Part model, mm, in its own coordinate system. Face numbers are marked on the shaded views. A direction names the side the tool comes from. Give positions to 0.01 mm unless a question says otherwise; leave off trailing zeros. Order: outer loops, then holes, each group sorted by start corner. A loop starts at its lowest first (then second) coordinate and runs counter-clockwise, first axis right, second up. Notation, with made-up numbers: (37.25, 53) - (84.25, 53) arc R23 cw to (84.25, 71) - close; hole circle Ø7 at (41, 11.5). An arc over 180 degrees is marked (long way). One line per item, written item: value.
```python
from build123d import *

# Parameters (mm, degrees)
BOSS_EXTRUDE1_DEPTH      = 30
SKETCH2_R                = 5
CUT_EXTRUDE1_DEPTH       = 30
BOSS_EXTRUDE2_DEPTH      = 10
BOSS_EXTRUDE2_DEPTH_BACK = 10
SKETCH4_W                = 159.060966422
SKETCH4_H                = 100
CUT_EXTRUDE2_DEPTH       = 55
CUT_EXTRUDE3_DEPTH       = 10
CUT_EXTRUDE3_DEPTH_BACK  = 5
SKETCH6_R                = 4.5
BOSS_EXTRUDE3_DEPTH      = 5


with BuildPart() as part:
    # Sketch1 → Boss-Extrude1 (new body)
    with BuildSketch(Plane(origin=(0, 0, 0), x_dir=(1, 0, 0), z_dir=(0, 1, 0))):
        with BuildLine():
            Line((2.5, 100), (0, 100))
            Line((0, 100), (0, 97.5))
            Line((0, 97.5), (0, 2.5))
            ThreePointArc((0, 2.5), (0.732233047, 0.732233047), (2.5, 0))
            Line((2.5, 0), (305, 0))
            ThreePointArc((305, 0), (315.606601718, 4.393398282), (320, 15))
            Line((320, 15), (320, 85))
            ThreePointArc((320, 85), (315.606601718, 95.606601718), (305, 100))
            Line((305, 100), (2.5, 100))
        make_face()
        with BuildLine():
            Line((20, 95), (300, 95))
            ThreePointArc((300, 95), (310.606601718, 90.606601718), (315, 80))
            Line((315, 80), (315, 20))
            ThreePointArc((315, 20), (310.606601718, 9.393398282), (300, 5))
            Line((300, 5), (20, 5))
            ThreePointArc((20, 5), (9.393398282, 9.393398282), (5, 20))
            Line((5, 20), (5, 80))
            ThreePointArc((5, 80), (9.393398282, 90.606601718), (20, 95))
        make_face(mode=Mode.SUBTRACT)
    extrude(amount=BOSS_EXTRUDE1_DEPTH)

    # Sketch2 → Cut-Extrude1 (cut)
    with BuildSketch(Plane(origin=(0, 0, 0), x_dir=(0, 0, -1), z_dir=(1, 0, 0))):
        with Locations((50, 3)):
            Circle(SKETCH2_R)
    extrude(amount=CUT_EXTRUDE1_DEPTH, mode=Mode.SUBTRACT)

    # Sketch3 → Boss-Extrude2 (add, two sides: drawn at the far end of the back side and taken through both)
    with BuildSketch(Plane(origin=(160, 0, 0), x_dir=(0, 0, -1), z_dir=(1, 0, 0)).offset(-BOSS_EXTRUDE2_DEPTH_BACK)):
        Polygon((5, 0), (5, 5), (7.5, 2.5), align=None)
        Polygon((95, 0), (95, 5), (92.5, 2.5), align=None)
    extrude(amount=BOSS_EXTRUDE2_DEPTH + BOSS_EXTRUDE2_DEPTH_BACK)

    # Sketch4 → Cut-Extrude2 (cut)
    with BuildSketch(Plane(origin=(0, 0, 0), x_dir=(1, 0, 0), z_dir=(0, 1, 0))):
        with Locations((249.530483211, 50)):
            Rectangle(SKETCH4_W, SKETCH4_H)
    extrude(amount=CUT_EXTRUDE2_DEPTH, mode=Mode.SUBTRACT)

    # Sketch5 → Cut-Extrude3 (cut, two sides: drawn at the far end of the back side and taken through both)
    with BuildSketch(Plane(origin=(160, 0, 0), x_dir=(0, 0, -1), z_dir=(1, 0, 0)).offset(-CUT_EXTRUDE3_DEPTH_BACK)):
        with BuildLine():
            ThreePointArc((3.5, 25), (3.207106781, 25.707106781), (2.5, 26))
            Line((2.5, 26), (2.5, 4))
            ThreePointArc((2.5, 4), (3.207106781, 4.292893219), (3.5, 5))
            Line((3.5, 5), (3.5, 25))
        make_face()
        with BuildLine():
            Line((2.5, 4), (2.5, 26))
            ThreePointArc((2.5, 26), (1.792893219, 25.707106781), (1.5, 25))
            Line((1.5, 25), (1.5, 5))
            ThreePointArc((1.5, 5), (1.792893219, 4.292893219), (2.5, 4))
        make_face()
        with BuildLine():
            ThreePointArc((98.5, 25), (98.207106781, 25.707106781), (97.5, 26))
            Line((97.5, 26), (97.5, 4))
            ThreePointArc((97.5, 4), (98.207106781, 4.292893219), (98.5, 5))
            Line((98.5, 5), (98.5, 25))
        make_face()
        with BuildLine():
            Line((97.5, 4), (97.5, 26))
            ThreePointArc((97.5, 26), (96.792893219, 25.707106781), (96.5, 25))
            Line((96.5, 25), (96.5, 5))
            ThreePointArc((96.5, 5), (96.792893219, 4.292893219), (97.5, 4))
        make_face()
    extrude(amount=CUT_EXTRUDE3_DEPTH + CUT_EXTRUDE3_DEPTH_BACK, mode=Mode.SUBTRACT)

    # Sketch6 → Boss-Extrude3 (add)
    with BuildSketch(Plane(origin=(0, 0, 0), x_dir=(0, 0, -1), z_dir=(1, 0, 0))):
        with Locations((50, 33)):
            Circle(SKETCH6_R)
    extrude(amount=BOSS_EXTRUDE3_DEPTH)


solid = part.part
```
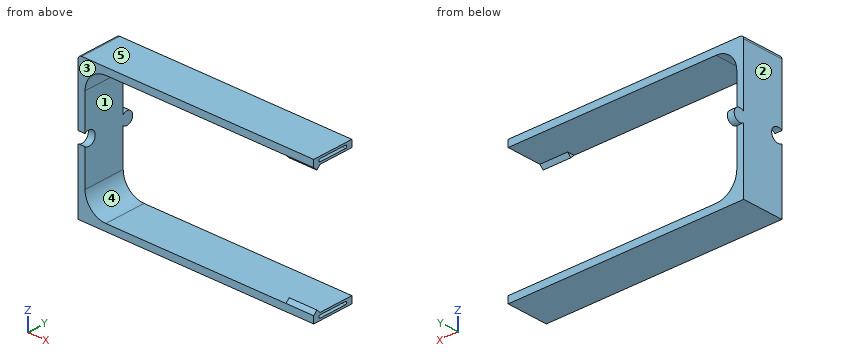
1) Cut at D-D, the plane z = -65.5. Give the cut face in (x, y).
Outcome:
outline: (0, 0) - (5, 0) - (5, 30) - (0, 30) - close
2) Cut at A-A, the plane x = 157.5. Give the cut face in (y, z), then the cut area to 3 significant figures.
Outcome:
outline: (0, -100) - (30, -100) - (30, -95) - (5, -95) - (2.5, -92.5) - (0, -95) - close; (0, -5) - (2.5, -7.5) - (5, -5) - (30, -5) - (30, 0) - (0, 0) - close; hole (5, -98.5) - (25, -98.5) arc R1 ccw to (25, -96.5) - (5, -96.5) arc R1 ccw to start; hole (5, -3.5) - (25, -3.5) arc R1 ccw to (25, -1.5) - (5, -1.5) arc R1 ccw to start
area: 226 mm^2
3) Cut at C-C, the plane y = 16.5. Give the cut face in (x, z), then the cut area to 3 significant figures.
Outcome:
outline: (0, -100) - (170, -100) - (170, -98.5) - (155, -98.5) - (155, -96.5) - (170, -96.5) - (170, -95) - (20, -95) arc R15 cw to (5, -80) - (5, -20) arc R15 cw to (20, -5) - (170, -5) - (170, -3.5) - (155, -3.5) - (155, -1.5) - (170, -1.5) - (170, 0) - (2.5, 0) arc R2.5 ccw to (0, -2.5) - close
area: 2,190 mm^2
4) Which spindle directions (+Z, -Z, +X, -X, +Y, -Y) get a long thin tool onto all of the face, cutting with end or side? Do the marked faces 1 and 2. Say none if no direction does.
Outcome:
face 1: +X, +Y, -Y
face 2: +Z, -Z, -X, +Y, -Y
5) Cut at B-B, the plane x = 123.5. Give the cut face in (y, z), then the cut area to 3 significant figures.
Outcome:
outline: (0, -100) - (30, -100) - (30, -95) - (0, -95) - close; (0, -5) - (30, -5) - (30, 0) - (0, 0) - close
area: 300 mm^2
6) Pin check, flat tips, straight feed: pin 1 (11 mm diameter, centred on y = 24, z = -41.5, fed in from +X); pin 2 (1.6 mm diameter, centred on y = 20, z = -2.5, fed in from +X). Stop position of each tip, or through.
Outcome:
pin 1: stops at x = 5
pin 2: stops at x = 155
7) Mould opens along Z. For the marked faces 3, 4 and 5 say: released by +Z, released by -Z, zero draft, split by the parting line, or undercut.
Outcome:
face 3: zero draft
face 4: undercut
face 5: released by +Z
8) Drill centre lines: line 1 along Z through (x, y) = (118.5, 5); line 2 along X through (y, z) = (8.5, -23); line 3 along Z through (x, y) = (3.1, 3). Where is each one in solid material? Low to high. Write a range as from..to.
Outcome:
line 1: z = -100..-95, -5..0
line 2: x = 0..5
line 3: z = -100..-55, -45..0
